Geometry: final body of the model. Coordinates: model frame, mm. A direction names the side the tool comes from. Round coordinates to 2 decimals unless told otherwise and drop trailing zeros. Write each loop counter-clockwise with the first axis right and the second up, starting at its lowest first coordinate (ties: lowest second). Pieces come first, ordered by that corner, then holes. Notation, with made-up numbers: (49, 20) -> (54, 20) arc R26 ccw to (54, 39) -> close; hole circle Ø11 at (81, 5.25). An arc over 180 degrees is marked (long way). One line per item, written item: value. Start each with the question number.
from build123d import *

# Parameters (mm, degrees)
NGULO_L_L2_5X2X0_25_1_DEPTH = 500
CROQUIS3_R                  = 4.7625
CORTAR_EXTRUIR1_DEPTH       = 6.35


with BuildPart() as part:
    # Sketch1 → Ángulo l L2.5X2X0.25(1) (new body)
    with BuildSketch(Plane.ZX):
        with BuildLine():
            Line((0, 0), (0, 63.5))
            Line((0, 63.5), (1.59258, 63.5))
            ThreePointArc((1.59258, 63.5), (4.956583943, 62.106583943), (6.35, 58.74258))
            Line((6.35, 58.74258), (6.35, 11.1125))
            ThreePointArc((6.35, 11.1125), (7.744903955, 7.744903955), (11.1125, 6.35))
            Line((11.1125, 6.35), (46.04258, 6.35))
            ThreePointArc((46.04258, 6.35), (49.406583943, 4.956583943), (50.8, 1.59258))
            Line((50.8, 1.59258), (50.8, 0))
            Line((50.8, 0), (0, 0))
        make_face()
    extrude(amount=NGULO_L_L2_5X2X0_25_1_DEPTH)

    # Croquis3 → Cortar-Extruir1 (cut)
    with BuildSketch(Plane.XY.offset(6.35)):
        with Locations((34.92754, 465)):
            Circle(CROQUIS3_R)
        with Locations((34.92754, 35)):
            Circle(CROQUIS3_R)
    extrude(amount=-CORTAR_EXTRUIR1_DEPTH, mode=Mode.SUBTRACT)


solid = part.part
(1) Section query C-C (z = 22). Output: boundary loops of the cut face in (x, y).
(2) Pin query (flat end, axial travel): pin 1 (12 mm diameter, centred on x = 14, z = 18.5, fed in from +Y); pin 2 (1 mm diameter, centred on x = 53.5, y = 397, fed in from +Z); pin 3 (3 mm diameter, centred on x = 40.5, y = 71.5, fed in from -Z); pin 4 (10 mm diameter, centred on y = 382, z = 32.5, fed in from +X). Return the tip coordinate at first contact, or that it passes through.
(3) Pull-direction query (Y, two-part tool) for faces 3 (the face through (34.308, 469.722, 3.219)), 4 (the face through (35, 246, 6.35)), 5 (the face through (20, 500, 5)), 6 (the face through (31.4, 38.2, 3.2)); classes: pulls with the +Y half, pulls with the -Y half, needs draft (parallel to the pull), parting line crosses it, or undercut.
(4) Line query: probe 1 along Z at (x, y) = (33.5, 269); probe 2 along X at (y, z) = (465, 4). Output: solid intervals per line, ascending.
(5) Set-up query: faces 1 (the face through (6.35, 246, 28)), 2 (the face through (20, 0, 5)). Return all of +Z, -Z, +X, -X, +Y, -Y with unobstructed straight access to the full face (end or side cutting, diameter ignored); none if empty.
Results list:
1. outline: (0, 0) -> (6.35, 0) -> (6.35, 500) -> (0, 500) -> close
2. pin 1: passes through
2. pin 2: stops at z = 6.35
2. pin 3: stops at z = 0
2. pin 4: stops at x = 6.35
3. face 3: undercut
3. face 4: needs draft
3. face 5: pulls with the +Y half
3. face 6: undercut
4. probe 1: z = 0 to 6.35
4. probe 2: x = 0 to 30.17, 39.69 to 62.85
5. face 1: +Z, +X, +Y, -Y
5. face 2: +Z, -Z, +X, -X, -Y
